from build123d import *

# Parameters (mm, degrees)
ESBO_O1_R                = 5
ESBO_O1_R_2              = 2.1
RESSALTO_EXTRUS_O1_DEPTH = 12
ESBO_O2_R                = 1.5
CORTE_EXTRUS_O1_DEPTH    = 10
RESSALTO_EXTRUS_O2_DEPTH = 5
ESBO_O4_R                = 1.5
CORTE_EXTRUS_O2_DEPTH    = 5
FILETE1_R                = 1
FILETE2_R                = 3


with BuildPart() as part:
    # Esboço1 → Ressalto-extrusão1 (new body)
    with BuildSketch(Plane(origin=(0, 0, 0), x_dir=(1, 0, 0), z_dir=(0, 1, 0))):
        with Locations(Location((0, 0, 0), (0, 0, 270))):
            Circle(ESBO_O1_R)
        with Locations(Location((0, 0, 0), (0, 0, 270))):
            Circle(ESBO_O1_R_2, mode=Mode.SUBTRACT)
    extrude(amount=RESSALTO_EXTRUS_O1_DEPTH)

    # Esboço2 → Corte-extrusão1 (cut)
    with BuildSketch(Plane.XY):
        with Locations(Location((0, 3, 0), (0, 0, 180))):
            Circle(ESBO_O2_R)
    extrude(amount=CORTE_EXTRUS_O1_DEPTH, mode=Mode.SUBTRACT)

    # Esboço3 → Ressalto-extrusão2 (add, symmetric)
    with BuildSketch(Plane.XY):
        Polygon((4.070319398, 10), (8.140638796, 17.05), (4.070319398, 24.1), (-4.070319398, 24.1), (-8.140638796, 17.05), (-4.070319398, 10), align=None)
        Polygon((2.33826859, 13), (4.67653718, 17.05), (2.33826859, 21.1), (-2.33826859, 21.1), (-4.67653718, 17.05), (-2.33826859, 13), align=None, mode=Mode.SUBTRACT)
    extrude(amount=RESSALTO_EXTRUS_O2_DEPTH, both=True)

    # Esboço4 → Corte-extrusão2 (cut)
    with BuildSketch(Plane(origin=(0, 24.1, 0), x_dir=(1, 0, 0), z_dir=(0, 1, 0))):
        with Locations(Location((0, 0, 0), (0, 0, 270))):
            Circle(ESBO_O4_R)
    extrude(amount=-CORTE_EXTRUS_O2_DEPTH, mode=Mode.SUBTRACT)

    # Filete1
    filete1_edges = [part.edges().sort_by_distance(p)[0] for p in [
        (0, 0, -5),
        (0, 13, -5),
        (3.507402885, 15.025, -5),
        (3.507402885, 19.075, -5),
        (0, 21.1, -5),
        (-3.507402885, 19.075, -5),
        (-3.507402885, 15.025, -5),
        (0, 13, 5),
        (3.507402885, 15.025, 5),
        (3.507402885, 19.075, 5),
        (0, 21.1, 5),
        (-3.507402885, 19.075, 5),
        (-3.507402885, 15.025, 5),
        (0, 0, -2.1),
    ]]
    fillet(filete1_edges, radius=FILETE1_R - 0.0001)  # a hair under: the kernel refuses the full size

    # Filete2
    filete2_edges = [part.edges().sort_by_distance(p)[0] for p in [
        (-4.070319398, 10, -3.95193836),
        (-4.070319398, 10, 3.95193836),
        (8.140638796, 17.05, 0),
        (4.070319398, 10, 3.95193836),
        (4.070319398, 10, -3.95193836),
        (4.070319398, 24.1, 0),
        (-4.070319398, 24.1, 0),
        (-8.140638796, 17.05, 0),
    ]]
    fillet(filete2_edges, radius=FILETE2_R)


solid = part.part
Geometry: final body of the model. Coordinates: model frame, mm. A direction names the side the tool comes from. Round coordinates to 2 decimals unless told otherwise and drop trailing zeros. Put each result on its own line as item: value. Start each with the question number.
Q1. Line query: probe 1 along Y at (x, z) = (0, 4); probe 2 along Z at (x, y) = (0, 7.25). Output: solid intervals per line, ascending.
Q2. Pull-direction query (X, two-part tool) for faces 4 (the flat face through (-2, 24.1, 0)), 5 (the flat face through (-6.12, 13.55, 0.07)), 6 (the flat face through (-3.491, 19.103, 0.056)); classes: +X half, -X half, draft (parallel to the pull), parting line (faces both ways), or undercut.
Q3. Reachability of faces 1 (the cylindrical face through (0.45, 22.62, 1.43)), 2 (the flat face through (0, 13, 0)), 3 (the cylindrical face through (-0.041, 21.401, 4.715)) from +Z, -Z, +X, -X, +Y, -Y: full face, straight path, thin tool, end or side. Return the list, or none.
Q4. First-contact query: pin 1 (4 mm diameter, centred on y = 5, z = 3.5, fed in from -X); pin 2 (5 mm diameter, centred on x = 5.5, z = -1.5, fed in from +Y); pin 3 (1.5 mm diameter, centred on x = 0, y = 21, fed in from -Z). Flat tips, straight axial feed; report the tip coordinate or a pass-through.
Ans:
1. probe 1: y = 0 to 1.5, 4.5 to 13, 21.1 to 24.1
1. probe 2: z = -5 to -2.1, 2.1 to 5
2. face 4: draft
2. face 5: -X half
2. face 6: undercut
3. face 1: +Y
3. face 2: +Z, -Z
3. face 3: +Z
4. pin 1: stops at x = -4.77
4. pin 2: stops at y = 24.03
4. pin 3: stops at z = -4.94
